Design review of the part built by this model. Coordinates are the model's own, in mm. Face numbers are marked on the shaded views. A direction names the side the tool comes from. Coordinates: 2 decimals unless noted, no trailing zeros. Write each loop counter-clockwise with the first axis right and the second up, starting at its lowest first coordinate (ties: lowest second). Pieces come first, ordered by that corner, then holes.
Q1. Add section D-D, the plane x = 58.5. Give the boundary of the cut face in (y, z), plus the area to 3 significant figures.
Q2. Add section C-C, the plane z = 15. Give the boundary of the cut face in (x, y).
Q3. To check wall thickness, follow probe 1 along Z at (x, y) = (118, 97); probe 2 along Y at (x, z) = (117.5, -21); probe 3 along Y at (x, z) = (33, 41.5). State the ranges of each line that lie inside material, in increasing order.
Q4. Machinability: for the marked faces 1, 2, 3 and 4, which of the approach directions +Z, -Z, +X, -X, +Y, -Y give a long, thin tool a straight path to every point of the face, cutting with its end or side? Answer none if there is none.
Q5. Add section B-B, the plane x = 119.5. Give the boundary of the cut face in (y, z).
Q6. The part is to be moulded in two halves that separate along Y. For the marked faces 5, 6, 7 and 8, say which applies: +Y half, -Y half, draft (parallel to the pull), parting line (faces both ways), or undercut.
Q7. Clearance check with flat-ended pins moving along their axes: pin 1 Ø3 at (x, z) = (94, 38) entering from +Y; pin 2 Ø9 at (x, y) = (103.5, -84) entering from +Z; pin 3 Ø10.5 at (x, y) = (12, -68.5) entering from +Z. State where each tip first meets the part, or that it passes through.
Q8. Add section A-A, the plane y = 37.5. Give the boundary of the cut face in (x, z) (3 decimals), plus the area to 3 significant figures.
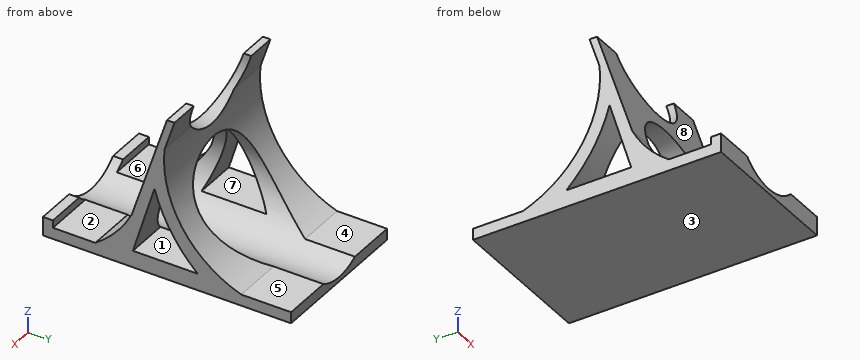
from build123d import *

# Parameters (mm, degrees)
F1_DEPTH = 127
F2_DEPTH = 127
F3_DEPTH = 127
F4_DEPTH = 127
F5_DEPTH = 127
F7_DEPTH = 114.3
F9_DEPTH = 215.9


# Not quite as in the source:
# - a feature names something its author has since deleted; it is built from what else it names


with BuildPart() as f1:
    # F0 (on Right) → F1 (new body)
    with BuildSketch(Plane.YZ):
        Polygon((-23.5780230826, -53.0224030194), (-17.2280230826, -53.0224030194), (15.5594434607, 47.8870429867), (23.9793931173, 73.8009834286), (17.6293931173, 73.8009834286), (-12.109174605, -17.7249168697), align=None)
        Polygon((-80.7280230826, -53.0224030194), (-80.7280230826, -62.5474030194), (122.4719769174, -62.5474030194), (122.4719769174, -53.0224030194), (80.3280323744, -53.0224030194), (-17.2280230826, -53.0224030194), (-23.5780230826, -53.0224030194), (-42.9109744728, -53.0224030194), (-78.7108764052, -53.0224030194), align=None)
    extrude(amount=F1_DEPTH)

    # F0 (on Right) → F2 (join)
    with BuildSketch(Plane.YZ):
        with BuildLine():
            Line((-17.2280230826, -53.0224030194), (80.3280323744, -53.0224030194))
            ThreePointArc((80.3280323744, -53.0224030194), (30.5185291001, -13.7520262922), (15.5594434607, 47.8870429867))
            Line((15.5594434607, 47.8870429867), (-17.2280230826, -53.0224030194))
        make_face()
        with BuildLine():
            Line((-11.1604323611, -48.4367646277), (7.0909718052, 11.3872801885))
            ThreePointArc((7.0909718052, 11.3872801885), (21.2331642185, -21.0320576084), (43.5937792063, -48.4367646277))
            Line((43.5937792063, -48.4367646277), (-11.1604323611, -48.4367646277))
        make_face(mode=Mode.SUBTRACT)
    extrude(amount=F2_DEPTH)

    # F0 (on Right) → F3 (cut)
    with BuildSketch(Plane.YZ):
        with BuildLine():
            ThreePointArc((43.5937792063, -48.4367646277), (21.2331642185, -21.0320576084), (7.0909718052, 11.3872801885))
            Line((7.0909718052, 11.3872801885), (-11.1604323611, -48.4367646277))
            Line((-11.1604323611, -48.4367646277), (43.5937792063, -48.4367646277))
        make_face()
    extrude(amount=-F3_DEPTH, mode=Mode.SUBTRACT)

    # F0 (on Right) → F4 (join)
    with BuildSketch(Plane.YZ):
        with BuildLine():
            ThreePointArc((-12.109174605, -17.7249168697), (-25.2658938129, -37.3320091963), (-42.9109744728, -53.0224030194))
            Line((-42.9109744728, -53.0224030194), (-23.5780230826, -53.0224030194))
            Line((-23.5780230826, -53.0224030194), (-12.109174605, -17.7249168697))
        make_face()
    extrude(amount=F4_DEPTH)

    # F0 (on Right) → F5 (join)
    with BuildSketch(Plane.YZ):
        Polygon((-87.1128812432, -62.5474030194), (-80.7280230826, -62.5474030194), (-80.7280230826, -53.0224030194), (-78.7108764052, -53.0224030194), (-78.7108764052, -46.6724030194), (-87.1128812432, -46.6724030194), align=None)
    extrude(amount=F5_DEPTH)

    # F6 (on face) → F7 (cut)
    with BuildSketch(Plane(origin=(0, -5.7436289571, 1.866218176), x_dir=(1, 0, 0), z_dir=(0, -0.9510565163, 0.3090169944))):
        with BuildLine():
            ThreePointArc((25.4, 75.6366882725), (63.5, 37.5366882725), (101.6, 75.6366882725))
            Line((101.6, 75.6366882725), (25.4, 75.6366882725))
        make_face()
        with BuildLine():
            Line((25.4, 75.6366882725), (101.6, 75.6366882725))
            ThreePointArc((101.6, 75.6366882725), (63.5, 113.7366882725), (25.4, 75.6366882725))
        make_face()
    extrude(amount=-F7_DEPTH, mode=Mode.SUBTRACT)

    # F8 (on face) → F9 (cut)
    with BuildSketch(Plane.XZ.offset(87.1128812432)):
        with BuildLine():
            Line((92.459596055, -46.6724030194), (34.2501482793, -46.6724030194))
            ThreePointArc((34.2501482793, -46.6724030194), (63.3548721671, -58.6806869), (92.459596055, -46.6724030194))
        make_face()
        with BuildLine():
            ThreePointArc((92.459596055, -46.6724030194), (101.4660457483, -33.2538436782), (104.6298721671, -17.4056869))
            ThreePointArc((104.6298721671, -17.4056869), (47.506715389, 20.7054866812), (34.2501482793, -46.6724030194))
            Line((34.2501482793, -46.6724030194), (92.459596055, -46.6724030194))
        make_face()
    extrude(amount=-F9_DEPTH, mode=Mode.SUBTRACT)


solid = f1.part
Here are the results:
1. outline: (-87.11, -62.55) - (122.47, -62.55) - (122.47, -58.39) - (-87.11, -58.39) - close; (1.31, 23.58) - (16.31, 23.58) arc R97.15 cw to (15.2, 34.88) - (5.96, 37.88) - close
1. area: 1,030 mm2
2. outline: (0, -1.48) - (37.79, -1.48) - (37.79, 18.07) - (0, 18.07) - close; (88.92, -1.48) - (127, -1.48) - (127, 18.07) - (88.92, 18.07) - close
3. probe 1: z = -62.55 to -53.02
3. probe 2: y = -13.83 to -2.79, 21.21 to 35.65
3. probe 3: y = 7.13 to 15.17
4. face 1: +X, -X
4. face 2: +Z, +X, -X
4. face 3: -Z, +X, -X, +Y, -Y
4. face 4: +Z, +X, -X, +Y
5. outline: (-87.11, -62.55) - (122.47, -62.55) - (122.47, -53.02) - (80.33, -53.02) arc R97.15 cw to (15.56, 47.89) - (23.98, 73.8) - (17.63, 73.8) - (-12.11, -17.72) arc R93.59 cw to (-42.91, -53.02) - (-78.71, -53.02) - (-78.71, -46.67) - (-87.11, -46.67) - close; hole (-11.16, -48.44) - (43.59, -48.44) arc R129.94 cw to (7.09, 11.39) - close
6. face 5: draft
6. face 6: undercut
6. face 7: undercut
6. face 8: -Y half
7. pin 1: stops at y = 15.15
7. pin 2: stops at z = -46.67
7. pin 3: stops at z = -53.02
8. outline: (0, -62.547) - (127, -62.547) - (127, -48.437) - (90.571, -48.437) arc R41.275 cw to (36.139, -48.437) - (0, -48.437) - close; (0, -42.372) - (30.487, -42.372) arc R41.275 cw to (22.502, -23.297) - (0, -23.297) - close; (96.223, -42.372) - (127, -42.372) - (127, -23.297) - (104.207, -23.297) arc R41.275 cw to start
8. area: 2,390 mm2
